from build123d import *

# Parameters (mm, degrees)
SKETCH2_W           = 46.482
SKETCH2_H           = 46.482
BOSS_EXTRUDE1_DEPTH = 66.04
SKETCH3_R           = 6.35
CUT_EXTRUDE1_DEPTH  = 12.7
SKETCH4_R           = 6.35
CUT_EXTRUDE2_DEPTH  = 12.7


with BuildPart() as part:
    # Sketch2 → Boss-Extrude1 (new body)
    with BuildSketch(Plane(origin=(0, 0, 0), x_dir=(1, 0, 0), z_dir=(0, 1, 0))):
        Rectangle(SKETCH2_W, SKETCH2_H)
    extrude(amount=BOSS_EXTRUDE1_DEPTH)

    # Sketch3 → Cut-Extrude1 (cut)
    with BuildSketch(Plane(origin=(0, 66.04, 0), x_dir=(1, 0, 0), z_dir=(0, 1, 0))):
        Circle(SKETCH3_R)
    extrude(amount=-CUT_EXTRUDE1_DEPTH, mode=Mode.SUBTRACT)

    # Sketch4 → Cut-Extrude2 (cut)
    with BuildSketch(Plane.XZ):
        Circle(SKETCH4_R)
    extrude(amount=-CUT_EXTRUDE2_DEPTH, mode=Mode.SUBTRACT)


solid = part.part
Geometry: final body of the model. Coordinates: model frame, mm. A direction names the side the tool comes from. Round coordinates to 2 decimals unless told otherwise and drop trailing zeros. Loops run counter-clockwise (first coordinate to the right, second up) from the corner with the lowest first, then second, coordinate; pieces in that order, holes last. Notation, with made-up numbers: M 54,51.25 L 109,51.25 A33 ccw 109,80.25 Z; hole C -23.5,-24.75 d3. An arc over 180 degrees is marked long. One line per question, with ' | ' between items.
(1) Cut plane A-A on y = 56. Return the cut outline in (x, z), plus the area to 3 significant figures.
Check result:
outline: M -23.24,-23.24 L 23.24,-23.24 L 23.24,23.24 L -23.24,23.24 Z; hole C 0,0 d12.7 | area: 2,030 mm2
(2) Contact query for a flat-ended pin moving along its axis: P1, Ø7.5, axis at x = 0, z = 0, coming from the -Y side. Output: stop coordinate, or through.
Check result:
P1: stops at y = 12.7
(3) Cut plane C-C on x = 0. Return the cut outline in (y, z), plus the area to 3 significant figures.
Check result:
outline: M 0,-23.24 L 66.04,-23.24 L 66.04,-6.35 L 53.34,-6.35 L 53.34,6.35 L 66.04,6.35 L 66.04,23.24 L 0,23.24 L 0,6.35 L 12.7,6.35 L 12.7,-6.35 L 0,-6.35 Z | area: 2,750 mm2
(4) Material intervals for line 1 along Z through (x, y) = (0, 63); line 2 along Z through (x, y) = (1.5, 57), sorted ascending. Write a range as from..to.
Check result:
line 1: z = -23.24..-6.35, 6.35..23.24 | line 2: z = -23.24..-6.17, 6.17..23.24
(5) Pull-direction query (X, two-part tool) for faces 4 (the cylindrical face through (-1.38, 6.26, -6.2)), 5 (the cylindrical face through (-1.38, 59.78, 6.2)), 6 (the flat face through (23.241, 33, 0)), 7 (the flat face through (0, 33, 23.241)); classes: +X half, -X half, draft (parallel to the pull), parting line (faces both ways), or undercut.
Check result:
face 4: undercut | face 5: undercut | face 6: +X half | face 7: draft
(6) Cut plane B-B on z = 0. Return the cut outline in (x, y), plus the area to 3 significant figures.
Check result:
outline: M -23.24,0 L -6.35,0 L -6.35,12.7 L 6.35,12.7 L 6.35,0 L 23.24,0 L 23.24,66.04 L 6.35,66.04 L 6.35,53.34 L -6.35,53.34 L -6.35,66.04 L -23.24,66.04 Z | area: 2,750 mm2
(7) Access query for faces 1 (the flat face through (0, 12.7, 0)), 2 (the flat face through (0, 53.34, 0)), 3 (the flat face through (5, 66.04, -5)). Directions: +Z, -Z, +X, -X, +Y, -Y. A direction counts if a zero-diameter tool reaches every point of the face in a straight line with its end or side. Return the directions, or none.
Check result:
face 1: -Y | face 2: +Y | face 3: +Z, -Z, +X, -X, +Y
